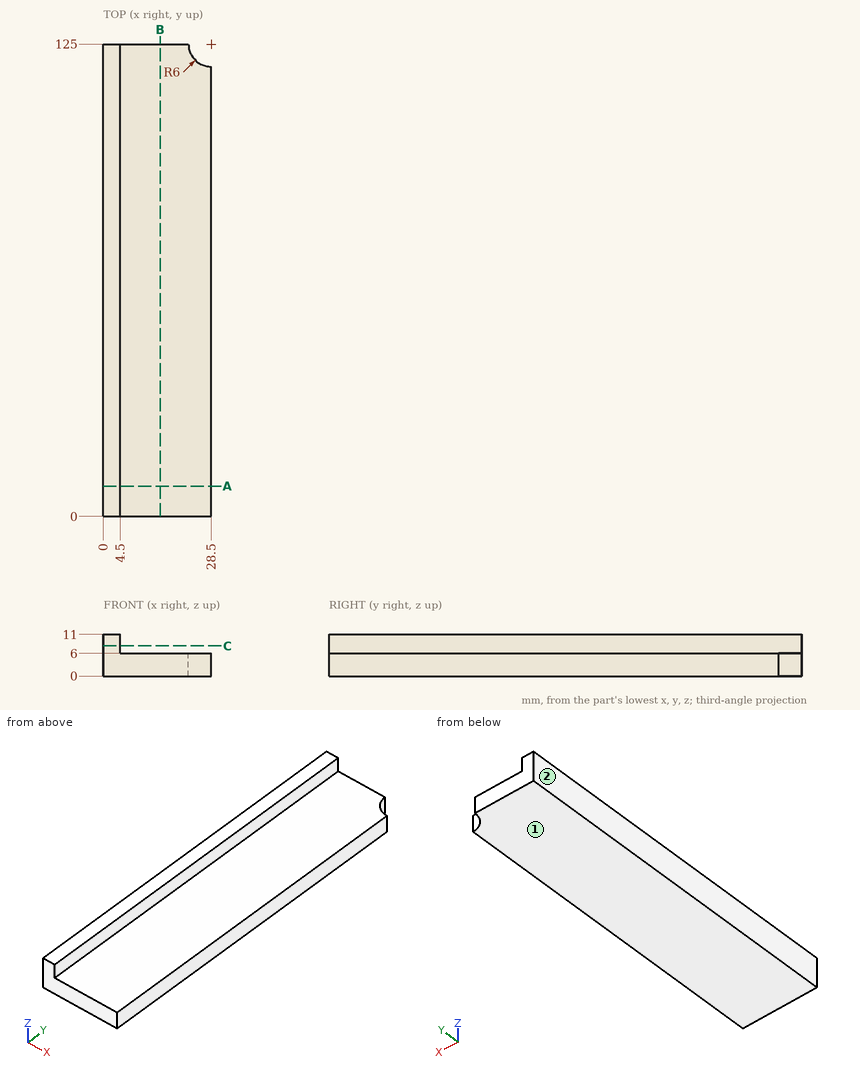
Study the drawing (mm; zero at the part's minimum x, y, z) and answer. Round coordinates to 2 decimals unless told otherwise and drop trailing zeros. Order: outer loops, then holes, each group sorted by start corner. A loop starts at its lowest first (then second) coordinate and runs counter-clockwise, first axis right, second up. Notation, with made-up numbers: (7.25, 60) - (22.25, 60) arc R22 cw to (22.25, 81) - close; hole circle Ø11 at (-26, 6.5). An arc over 180 degrees is marked (long way). Use one line per item in the form item = value. Start each with the question number.
(1) The part is cut by section A-A (y = 8). Give the vertices of the cut face in (x, z).
(2) The part is cut by section B-B (x = 15). Give the vertices of the cut face in (y, z), then the cut area to 3 significant figures.
(3) Find the intervals of material crossed by line 1 along X through (y, z) = (23, 8.5); line 2 along Z through (x, y) = (13.75, 63); line 3 along Y through (x, z) = (25, 4), in increasing order. Write a range as from..to.
(4) Determine the mould class of the marked faces 1 and 2 for opening direction X: +X half, -X half, draft (parallel to the pull), parting line (faces both ways), or undercut.
(5) The part is cut by section C-C (z = 8). Give the vertices of the cut face in (x, y), then the cut area to 4 significant figures.
(6) Flat-ended cylindrical pins translate along their axes: pin 1 Ø5.5 at (y, z) = (63.5, 9) entering from +X; pin 2 Ø12 at (x, y) = (14.5, 53.5) entering from +Z; pin 3 Ø1.5 at (x, y) = (12.5, 72.5) entering from -Z. Find the tip coordinate at first contact, or state that the pin passes through.
Checked values:
q1.outline = (0, 0) - (28.5, 0) - (28.5, 6) - (4.5, 6) - (4.5, 11) - (0, 11) - close
q2.outline = (0, 0) - (125, 0) - (125, 6) - (0, 6) - close
q2.area = 750 mm^2
q3.line_1 = 0..4.5
q3.line_2 = 0..6
q3.line_3 = 0..120.13
q4.face_1 = draft
q4.face_2 = -X half
q5.outline = (0, 0) - (4.5, 0) - (4.5, 125) - (0, 125) - close
q5.area = 562.5 mm^2
q6.pin_1 = 4.5
q6.pin_2 = 6
q6.pin_3 = 0
